Part print with two shaded views. Sizes in mm from the minimum x, y, z corner. Round coordinates to 2 decimals unless told otherwise and drop trailing zeros. Write each loop counter-clockwise with the first axis right and the second up, starting at its lowest first coordinate (ties: lowest second). Pieces come first, ordered by that corner, then holes. Notation, with made-up numbers: (-33.75, 19.25) -> (4.25, 19.25) arc R33 cw to (4.25, 53.25) -> close; hole circle Ø9 at (17.25, 68.25). An arc over 180 degrees is marked (long way). Return JSON: item names as keys, results as strings.
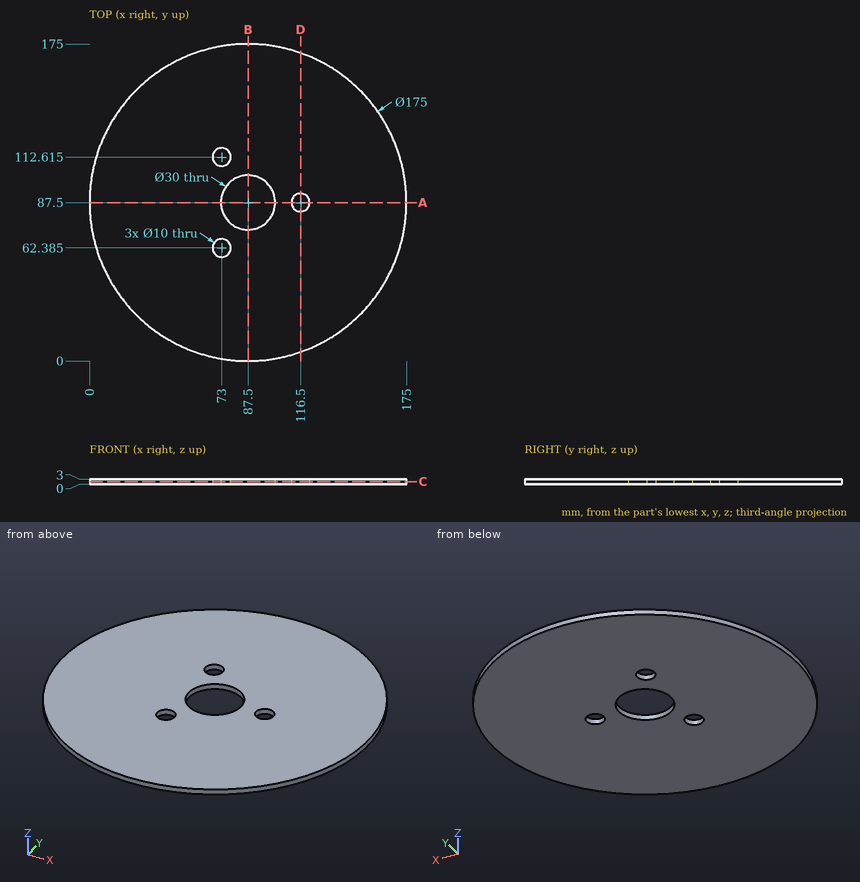
Q1. Saw through at B-B on x = 87.5. List the corners of the cut face in (y, z).
Verdict:
{"outline": "(0, 0) -> (72.5, 0) -> (72.5, 3) -> (0, 3) -> close; (102.5, 0) -> (175, 0) -> (175, 3) -> (102.5, 3) -> close"}
Q2. Saw through at A-A on y = 87.5. List the corners of the cut face in (x, z).
Verdict:
{"outline": "(0, 0) -> (72.5, 0) -> (72.5, 3) -> (0, 3) -> close; (102.5, 0) -> (111.5, 0) -> (111.5, 3) -> (102.5, 3) -> close; (121.5, 0) -> (175, 0) -> (175, 3) -> (121.5, 3) -> close"}
Q3. Wall check: L1, parallel to Y at x = 121, z = 1.8 (1 decimal); L2, parallel to X at y = 86, z = 0.2 (1 decimal); L3, parallel to Y at x = 116.5, z = 1.35 (1 decimal). Give the ranges that are in metal, low to high.
Verdict:
{"L1": "y = 6.7 to 85.3, 89.7 to 168.3", "L2": "x = 0 to 72.6, 102.4 to 111.7, 121.3 to 175", "L3": "y = 4.9 to 82.5, 92.5 to 170.1"}
Q4. Saw through at C-C on z = 1.6. List the corners of the cut face in (x, y) (1 decimal).
Verdict:
{"outline": "circle Ø175 at (87.5, 87.5); hole circle Ø10 at (73, 62.4); hole circle Ø10 at (73, 112.6); hole circle Ø30 at (87.5, 87.5); hole circle Ø10 at (116.5, 87.5)"}
Q5. Saw through at D-D on x = 116.5. List the corners of the cut face in (y, z) (1 decimal), then the cut area to 3 significant figures.
Verdict:
{"outline": "(4.9, 0) -> (82.5, 0) -> (82.5, 3) -> (4.9, 3) -> close; (92.5, 0) -> (170.1, 0) -> (170.1, 3) -> (92.5, 3) -> close", "area": "465 mm²"}
Q6. Pin check, flat tips, straight feed: pin 1 Ø1 at (y, z) = (93.5, 1.5) entering from -X; pin 2 Ø1 at (x, z) = (149, 2) entering from -Y. Stop position of each tip, or through.
Verdict:
{"pin 1": "stops at x = 0.17", "pin 2": "stops at y = 24.77"}
